Autodesk Fusion 360 part; units mm, degrees
sketch "Sketch1" plane through (0, 0, 0) normal (0, 0, 1) x (1, 0, 0)
  line L0 (67, 37) -> (-67, 37)
  line L1 (-67, 37) -> (-67, -37)
  line L2 (-67, -37) -> (67, -37)
  line L3 (67, -37) -> (67, 37)
  line L4 (67, 37) -> (-67, -37) construction
  line L5 (-67, 37) -> (67, -37) construction
  line L6 (70, 40) -> (-70, 40)
  line L7 (-70, 40) -> (-70, -40)
  line L8 (-70, -40) -> (70, -40)
  line L9 (70, -40) -> (70, 40)
  line L10 (70, 40) -> (-70, -40) construction
  line L11 (-70, 40) -> (70, -40) construction
  dimension "d1" = 3
  dimension "d2" = 3
  dimension "d3" = 140
  dimension "d4" = 80
extrude "Extrude1" add sketch "Sketch1" along normal blind 45
sketch "Sketch2" plane through (0, 0, 0) normal (0, 0, 1) x (1, 0, 0)
  line L0 (-67, 37) -> (67, 37)
  line L1 (67, 37) -> (67, -37)
  line L2 (67, -37) -> (-67, -37)
  line L3 (-67, -37) -> (-67, 37)
  point P0 (-67, 37)
  point P1 (67, -37)
extrude "Extrude2" add sketch "Sketch2" along normal blind 3
sketch "Sketch3" plane through (0, 0, 3) normal (0, 0, 1) x (-1, 0, 0)
  line L0 (67, 37) -> (-67, 37)
  line L1 (-67, 37) -> (-67, -37)
  line L2 (-67, -37) -> (67, -37)
  line L3 (67, -37) -> (67, 37)
  line L4 (57, -37) -> (67, -27)
  line L5 (67, -27) -> (67, -37)
  line L6 (57, -37) -> (67, -37)
  dimension "d11" = 10
  dimension "d12" = 10
extrude "Extrude3" add sketch "Sketch3" along normal up to surface (42 mm away) contours L2 L3 L4 L5 L6
sketch "Sketch5" plane through (0, 0, 45) normal (0, 0, 1) x (-1, 0, 0)
  line L0 (-67, -37) -> (-67, 37)
  line L1 (-67, 37) -> (67, 37)
  line L2 (67, 37) -> (67, -27)
  line L3 (67, -27) -> (57, -37)
  line L4 (57, -37) -> (-67, -37)
  line L5 (-70, 40) -> (-70, -40)
  line L6 (-70, -40) -> (70, -40)
  line L7 (70, -40) -> (70, 40)
  line L8 (70, 40) -> (-70, 40)
  circle A0 centre (65, -35) radius 1.5
  line L9 (0, -1.75) -> (0, -22.5)
  line L10 (-1.75, 0) -> (-22.5, 0)
  dimension "d18" = 3
  dimension "d19" = 65
  dimension "d20" = 35
extrude "Extrude5" cut sketch "Sketch5" against normal blind 20 contours A0
mirror "Mirror1" about plane through (0, 0, 0) normal (1, 0, 0) of "Extrude3", "Extrude5"
mirror "Mirror2" about plane through (0, 0, 0) normal (0, 1, 0) of "Mirror1", "Extrude5", "Extrude3"
sketch "Sketch6" plane through (67, 0, 0) normal (-1, 0, 0) x (0, -1, 0)
  line L0 (27, 3) -> (27, 45)
  line L1 (27, 45) -> (-27, 45)
  line L2 (-27, 45) -> (-27, 3)
  line L3 (-27, 3) -> (27, 3)
  line L4 (7.5, 3) -> (-7.5, 3)
  line L5 (-7.5, 3) -> (-7.5, 13)
  line L6 (-7.5, 13) -> (7.5, 13)
  line L7 (7.5, 13) -> (7.5, 3)
  line L8 (7.5, 3) -> (-7.5, 13) construction
  line L9 (-7.5, 3) -> (7.5, 13) construction
  line L10 (-27, 15.2846) -> (0, 15.2846) construction
  line L11 (0, 15.2846) -> (27, 15.2846) construction
  circle A0 centre (-4, 17) radius 1.5
  line L12 (0, 2.5) -> (0, 20)
  circle A1 centre (4, 17) radius 1.5
  point P0 (0, 8)
  dimension "d27" = 10
  dimension "d28" = 15
  dimension "d29" = 3
  dimension "d30" = 4
  dimension "d31" = 4
extrude "Extrude6" cut sketch "Sketch6" along normal mid plane 20 contours L3 L4 L6 L7 L12 | L3 L4 L5 L6 L12 | A0 | A1
fillet "Fillet1" radius 2 4 edges at (70, -40, 22.5) (70, 40, 22.5) (-70, 40, 22.5) (-70, -40, 22.5)
fillet "Fillet2" radius 1 5 edges at (70, 0, 13) (70, -7.5, 8) (70, 7.5, 8) (70, 5.3985, 16.4576) (67, 5.3985, 17.5424) 1 faces at (68, -5.4925, 16.8506)
Check sheet for the modelled part. Datum: model origin and axes. Units: mm. A direction names the side the tool comes from. Coordinates: 2 decimals unless noted, no trailing zeros. Write each loop counter-clockwise with the first axis right and the second up, starting at its lowest first coordinate (ties: lowest second). Pieces come first, ordered by that corner, then holes. Notation, with made-up numbers: M -0.75,75.5 L 46.25,75.5 A15 ccw 46.25,83.5 Z; hole C 27,43 d9. An arc over 180 degrees is marked long. Write item = value, one per line. Start each with the question number.
1. Sectioned sample at B-B (z = 27.5). Record the cut outline in (x, y).
2. Thickness scan on probe 1 along X at (y, z) = (17, 15); probe 2 along Y at (x, z) = (-49, 17.5); probe 3 along Y at (x, z) = (65, 35.5). Record the ranges inside material, lowest first.
3. Mould release check, pull along Y, two halves, no side actions. Record for faces 4 (the flat face through (-1, -40, 22)), 5 (the flat face through (-67, 0, 24)), 6 (the flat face through (-1, 1, 0)), 7 (the flat face through (1, 40, 22)): pulls with the +Y half, pulls with the -Y half, needs draft (parallel to the pull), parting line crosses it, or undercut.
4. Go/stop test with a flat-tipped pin: pin 1 (12 mm diameter, centred on x = 44.5, y = -13.5, fed in from +Z). Record where the tip stops, or that it passes through.
5. Sectioned sample at D-D (z = 10.5). Record the cut outline in (x, y), then the cut area to 3 significant figures.
6. Sectioned sample at C-C (y = 35). Record the cut outline in (x, z), then the cut area to 3 significant figures.
7. Sectioned sample at A-A (y = 4). Record the cut outline in (x, z).
8. Tool access check on faces 1 (the cylindrical face through (68.493, -4.806, 18.265)), 2 (the flat face through (70, -1, 22)), 3 (the flat face through (65, -35, 25)). Record the directions out of +Z, -Z, +X, -X, +Y, -Y that give a thin tool (end or side, any length) a straight path to the whole face; none if there is none.
The answers:
q1.outline = M -70,-38 A2 ccw -68,-40 L 68,-40 A2 ccw 70,-38 L 70,38 A2 ccw 68,40 L -68,40 A2 ccw -70,38 Z; hole M -67,-27 L -57,-37 L 57,-37 L 67,-27 L 67,27 L 57,37 L -57,37 L -67,27 Z; hole C -65,35 d3; hole C 65,-35 d3; hole C 65,35 d3
q2.probe_1 = -70 to -67, 67 to 70
q2.probe_2 = -40 to -37, 37 to 40
q2.probe_3 = -40 to -36.5, -33.5 to -29, 29 to 33.5, 36.5 to 40
q3.face_4 = pulls with the -Y half
q3.face_5 = undercut
q3.face_6 = needs draft
q3.face_7 = pulls with the +Y half
q4.pin_1 = 3
q5.outline = M -70,-38 A2 ccw -68,-40 L 68,-40 A2 ccw 70,-38 L 70,-8.5 A1 ccw 69,-7.5 L 67,-7.5 L 67,-27 L 57,-37 L -57,-37 L -67,-27 L -67,27 L -57,37 L 57,37 L 67,27 L 67,7.5 L 69,7.5 A1 ccw 70,8.5 L 70,38 A2 ccw 68,40 L -68,40 A2 ccw -70,38 Z
q5.area = 1,440 mm²
q6.outline = M -70,0 L 70,0 L 70,45 L 66.5,45 L 66.5,25 L 63.5,25 L 63.5,45 L 59,45 L 59,3 L -59,3 L -59,45 L -63.5,45 L -63.5,25 L -66.5,25 L -66.5,45 L -70,45 Z
q6.area = 1,220 mm²
q7.outline = M -70,0 L 70,0 L 70,3 L -67,3 L -67,45 L -70,45 Z; M 67,13 L 69,13 A1 ccw 70,14 L 70,14.5 A1 ccw 69,15.5 L 68,15.5 A1 ccw 67,14.5 Z; M 67,19.5 A1 ccw 68,18.5 L 69,18.5 A1 ccw 70,19.5 L 70,45 L 67,45 Z
q8.face_1 = +X
q8.face_2 = +Z, -Z, +X, +Y, -Y
q8.face_3 = +Z
